Check sheet for the modelled part. Datum: model origin and axes. Units: mm. A direction names the side the tool comes from. Coordinates: 2 decimals unless noted, no trailing zeros. Write each loop counter-clockwise with the first axis right and the second up, starting at its lowest first coordinate (ties: lowest second). Pieces come first, ordered by that corner, then holes. Notation, with made-up numbers: M 58,33.5 L 87,33.5 A13 cw 87,57.5 Z; hole C 13.5,11.25 d6. An arc over 180 degrees is marked long. Answer as CSV lines item,"result". Start each with the question number.
Q1. Mould release check, pull along X, two halves, no side actions. Record for faces 3 (the flat face through (-12.864, 14.957, 4.563)), 4 (the cylindrical face through (-12.604, 5.916, 9.523)), 5 (the flat face through (-14, 18, 11)), 6 (the flat face through (-14, 12, 11)): pulls with the +X half, pulls with the -X half, needs draft (parallel to the pull), parting line crosses it, or undercut.
Q2. Sectioned sample at A-A, the plane y = 2.5. Record the cut outline in (x, z).
Q3. Access from +Z, -Z, +X, -X, +Y, -Y to the whole of each face (thin tool, end or side, straight path). Record for faces 1 (the flat face through (-18.293, 14.957, 15.265)), 2 (the flat face through (-20, 12, 6)).
Q4. Thickness scan on line 1 along X through (y, z) = (10.75, 10.25); line 2 along X through (y, z) = (5.5, 12.5); line 3 along Y through (x, z) = (-17.75, 11.5). Record the ranges inside material, lowest first. Write a range as from..to.
Q5. Depth check by flat-ended pin: pin 1 Ø5 at (y, z) = (7, 6) entering from -X; pin 2 Ø3 at (y, z) = (6.5, 15.5) entering from -X; pin 3 Ø1 at (x, y) = (-19.5, 8) entering from +Z. Enter the tip coordinate at first touch or a pass-through.
Q6. Sectioned sample at B-B, the plane y = 5.25. Record the cut outline in (x, z).
from build123d import *

# Parameters (mm, degrees)
SKETCH1_R           = 5.5
SKETCH1_R_2         = 3
BOSS_EXTRUDE1_DEPTH = 12
BOSS_EXTRUDE2_DEPTH = 6
CUT_EXTRUDE1_DEPTH  = 17
CUT_EXTRUDE4_DEPTH  = 22


with BuildPart() as part:
    # Sketch1 → Boss-Extrude1 (new body)
    with BuildSketch(Plane(origin=(0, 0, 0), x_dir=(1, 0, 0), z_dir=(0, 1, 0))):
        with Locations(Location((-15.57885573, -9.913817283, 0), (0, 0, 270))):
            Circle(SKETCH1_R)
        with Locations(Location((-15.57885573, -9.913817283, 0), (0, 0, 270))):
            Circle(SKETCH1_R_2, mode=Mode.SUBTRACT)
    extrude(amount=BOSS_EXTRUDE1_DEPTH)

    # Sketch2 → Boss-Extrude2 (add)
    with BuildSketch(Plane(origin=(0, 12, 0), x_dir=(1, 0, 0), z_dir=(0, 1, 0))):
        Polygon((-15.148097749, -16.828616453), (-9.375084996, -12.998169513), (-9.805842977, -6.083370343), (-16.009613711, -2.999018113), (-21.782626464, -6.829465052), (-21.351868483, -13.744264222), align=None)
    extrude(amount=BOSS_EXTRUDE2_DEPTH)

    # Sketch3 → Cut-Extrude1 (cut)
    with BuildSketch(Plane(origin=(0, 18, 0), x_dir=(1, 0, 0), z_dir=(0, 1, 0))):
        with BuildLine():
            ThreePointArc((-13.95385573, -9.913817283), (-14.810518846, -8.481936201), (-16.477281493, -8.55976553))
            Line((-16.477281493, -8.55976553), (-14.680429966, -11.267869035))
            ThreePointArc((-14.680429966, -11.267869035), (-14.146974648, -10.682154166), (-13.95385573, -9.913817283))
        make_face()
        with BuildLine():
            Line((-14.680429966, -11.267869035), (-16.477281493, -8.55976553))
            ThreePointArc((-16.477281493, -8.55976553), (-16.932907482, -10.812243046), (-14.680429966, -11.267869035))
        make_face()
    extrude(amount=-CUT_EXTRUDE1_DEPTH, mode=Mode.SUBTRACT)

    # Sketch5 → Cut-Revolve1 (revolve, cut)
    with BuildSketch(Plane(origin=(-16.133827612, 0, 1.005058114), x_dir=(0.06217455908352037, 0, 0.9980652905510591), z_dir=(-0.9980652905510591, 0, 0.06217455908352037)), mode=Mode.PRIVATE) as cut_revolve1_sk:
        with BuildLine():
            Line((15.854231671, 18), (15.854231671, 17))
            ThreePointArc((15.854231671, 17), (15.561338452, 17.707106781), (14.854231671, 18))
            Line((14.854231671, 18), (15.854231671, 18))
        make_face()
    revolve(cut_revolve1_sk.sketch.rotate(Axis((-15.57885573, 18, 9.913817283), (0, 1, 0)), 356.435361028), axis=Axis((-15.57885573, 18, 9.913817283), (0, 1, 0)), mode=Mode.SUBTRACT)

    # Sketch6 → Cut-Extrude4 (cut)
    with BuildSketch(Plane(origin=(-10.145435869, 0, 0.632010759), x_dir=(-0.06217455908352025, 0, -0.9980652905510591), z_dir=(0.9980652905510591, 0, -0.06217455908352025))):
        with BuildLine():
            ThreePointArc((-8.926028441, 4.5), (-10.176028441, 3.25), (-8.926028441, 2))
            Line((-8.926028441, 2), (-8.926028441, 4.5))
        make_face()
        with BuildLine():
            Line((-8.926028441, 4.5), (-8.926028441, 2))
            ThreePointArc((-8.926028441, 2), (-8.042144964, 2.366116524), (-7.676028441, 3.25))
            ThreePointArc((-7.676028441, 3.25), (-8.042144964, 4.133883476), (-8.926028441, 4.5))
        make_face()
    extrude(amount=-CUT_EXTRUDE4_DEPTH, mode=Mode.SUBTRACT)


solid = part.part
Output:
1,face 3,"pulls with the +X half"
1,face 4,"undercut"
1,face 5,"needs draft"
1,face 6,"undercut"
2,outline,"M -21.04,9.25 A5.5 ccw -10.24,8.58 L -12.82,8.74 A3 cw -18.46,9.09 Z; M -20.91,11.25 L -18.34,11.09 A3 cw -12.69,10.74 L -10.12,10.58 A5.5 ccw Z"
3,face 1,"+Z, -X, +Y, -Y"
3,face 2,"-Y"
4,line 1,"x = -21.07..-18.56, -12.6..-10.09"
4,line 2,"x = -20.43..-17.1, -14.06..-10.72"
4,line 3,"y = 12..18"
5,pin 1,"stops at x = -20.89"
5,pin 2,"stops at x = -19.26"
5,pin 3,"stops at z = 14.22"
6,outline,"C -15.58,9.91 d11; hole C -15.58,9.91 d6"
